CAD build for the part. Positions are in the model's coordinates, mm. Round coordinates to 2 decimals unless told otherwise and drop trailing zeros. Loops run counter-clockwise (first coordinate to the right, second up) from the corner with the lowest first, then second, coordinate; pieces in that order, holes last.
```python
from build123d import *

# Parameters (mm, degrees)
BOSS_EXTRUDE1_DEPTH                            = 6.35
M5_CLEARANCE_HOLE1_D                           = 5.5
M5_CLEARANCE_HOLE1_CSINK_D                     = 5.55
M5_CLEARANCE_HOLE1_CSINK_ANGLE                 = 90
SKETCH5_R                                      = 7.5
CUT_EXTRUDE1_DEPTH                             = 81.928436696
CSK_FOR_M8_FLAT_HEAD_MACHINE_SCREW1_AT_2_COUNT = 2
CSK_FOR_M8_FLAT_HEAD_MACHINE_SCREW1_AT_2_PITCH = 25
FILLET1_R                                      = 25


with BuildPart() as part:
    # Sketch1 → Boss-Extrude1 (new body)
    with BuildSketch(Plane(origin=(0, 0, 0), x_dir=(1, 0, 0), z_dir=(0, 1, 0))):
        with BuildLine():
            Line((-12.5, -72.691742077), (12.5, -72.691742077))
            Line((12.5, -72.691742077), (12.5, -32.691742077))
            ThreePointArc((12.5, -32.691742077), (0, 35), (-12.5, -32.691742077))
            Line((-12.5, -32.691742077), (-12.5, -72.691742077))
        make_face()
    extrude(amount=BOSS_EXTRUDE1_DEPTH)

    # M5 Clearance Hole1 (through all)
    with Locations(Plane(origin=(0, 0, 0), x_dir=(-1, 0, 0), z_dir=(0, -1, 0))):
        with Locations((0, 17.5), (12.374368671, 12.374368671), (17.5, 0), (12.374368671, -12.374368671), (0, -17.5), (-12.374368671, -12.374368671), (-17.5, 0), (-12.374368671, 12.374368671)):
            CounterSinkHole(M5_CLEARANCE_HOLE1_D / 2, M5_CLEARANCE_HOLE1_CSINK_D / 2, counter_sink_angle=M5_CLEARANCE_HOLE1_CSINK_ANGLE)

    # Sketch5 → Cut-Extrude1 (cut, through all)
    with BuildSketch(Plane.XZ):
        with Locations(Location((0, 0, 0), (0, 0, 270))):
            Circle(SKETCH5_R)
    extrude(amount=-CUT_EXTRUDE1_DEPTH, mode=Mode.SUBTRACT)

    # Sketch8 → CSK for M8 Flat Head Machine Screw1 (revolve, cut)
    with BuildSketch(Plane(origin=(0, 0, 37.691742077), x_dir=(0, 0, -1), z_dir=(1, 0, 0))):
        Polygon((0, 0), (0, 6.35), (5, 6.35), (5, 3.65), (8.65, 0), align=None)
    csk_for_m8_flat_head_machine_screw1 = revolve(axis=Axis((0, -6.35, 37.691742077), (0, 1, 0)), mode=Mode.SUBTRACT)

    # CSK for M8 Flat Head Machine Screw1 at 2: CSK for M8 Flat Head Machine Screw1 ×2
    with Locations(*[(0, 0, i * CSK_FOR_M8_FLAT_HEAD_MACHINE_SCREW1_AT_2_PITCH) for i in range(1, CSK_FOR_M8_FLAT_HEAD_MACHINE_SCREW1_AT_2_COUNT)]):
        add(csk_for_m8_flat_head_machine_screw1, mode=Mode.SUBTRACT)

    # Fillet1
    fillet1_edges = [part.edges().sort_by_distance(p)[0] for p in [
        (-12.5, 3.175, 32.691742077),
        (12.5, 3.175, 32.691742077),
    ]]
    fillet(fillet1_edges, radius=FILLET1_R)


solid = part.part
```
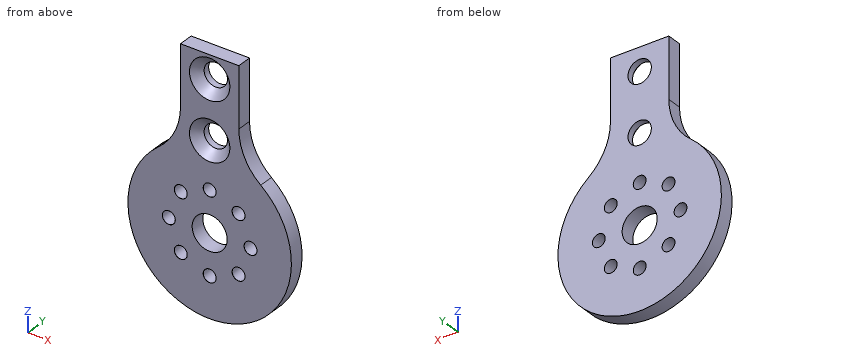
Item 1: Cut at A-A, the plane z = 0. Give the cut face in (x, y) (3 decimals).
Answers follow:
outline: (-35, 0) - (-20.275, 0) - (-20.25, 0.025) - (-20.25, 6.35) - (-35, 6.35) - close; (-14.75, 0.025) - (-14.725, 0) - (-7.5, 0) - (-7.5, 6.35) - (-14.75, 6.35) - close; (7.5, 0) - (14.725, 0) - (14.75, 0.025) - (14.75, 6.35) - (7.5, 6.35) - close; (20.25, 0.025) - (20.275, 0) - (35, 0) - (35, 6.35) - (20.25, 6.35) - close
Item 2: Probe line 1 (Z direction, x = 2, y = 6.25); line 2 (X direction, y = 2, z = 12); line 3 (Z direction, x = 5, y = 2.75). List the from-to ranges inside material, lowest first.
Answers follow:
line 1: z = -34.94 to -19.39, -15.61 to -7.23, 7.23 to 15.61, 19.39 to 33.11, 42.27 to 58.11, 67.27 to 72.69
line 2: x = -32.88 to -15.1, -9.65 to 9.65, 15.1 to 32.88
line 3: z = -34.64 to -5.59, 5.59 to 34.56, 40.82 to 59.56, 65.82 to 72.69
Item 3: Flat gauge pins, fed straight in: P1, Ø4, axis at x = 23, z = 8, coming from the -Y side; P2, Ø2, axis at y = 3, z = -3.5, coming from the +X side; P3, Ø1, axis at y = 2, z = 24.5, coming from the -X side. Where does each tip first touch, or does it go through?
Answers follow:
P1: stops at y = 0
P2: stops at x = 34.91
P3: stops at x = -25.48
Item 4: Cut at C-C, the plane z = 17.5. Give the cut face in (x, y) (3 decimals), plus the area to 3 significant figures.
Answers follow:
outline: (-30.311, 0) - (-2.775, 0) - (-2.75, 0.025) - (-2.75, 6.35) - (-30.311, 6.35) - close; (2.75, 0.025) - (2.775, 0) - (30.311, 0) - (30.311, 6.35) - (2.75, 6.35) - close
area: 350 mm2
Item 5: Cut at B-B, the plane x = 0. State how many separate pieces and enclosed holes the cut face has, plus the area to 3 significant figures.
Answers follow:
separate pieces: 6
enclosed holes: 0
area: 365 mm2
Item 6: Cut at D-D, the plane x = -17.5. Give the cut face in (y, z) (3 decimals).
Answers follow:
outline: (0, -30.311) - (6.35, -30.311) - (6.35, -2.75) - (0.025, -2.75) - (0, -2.775) - close; (0, 2.775) - (0.025, 2.75) - (6.35, 2.75) - (6.35, 31.837) - (0, 31.837) - close
